Check sheet for the drawn part. Datum: minimum x, y, z corner. Units: mm. A direction names the side the tool comes from. Round coordinates to 2 decimals unless told otherwise and drop trailing zeros. Write each loop counter-clockwise with the first axis right and the second up, starting at its lowest first coordinate (ties: lowest second). Pieces come first, ordered by that corner, then holes. Notation, with made-up numbers: (14, 28.5) -> (37, 28.5) arc R23 ccw to (37, 57.5) -> close; hole circle Ø7 at (-12.75, 62). An arc over 180 degrees is marked (long way). Use CSV: the item, a comma, the result in double quotes.
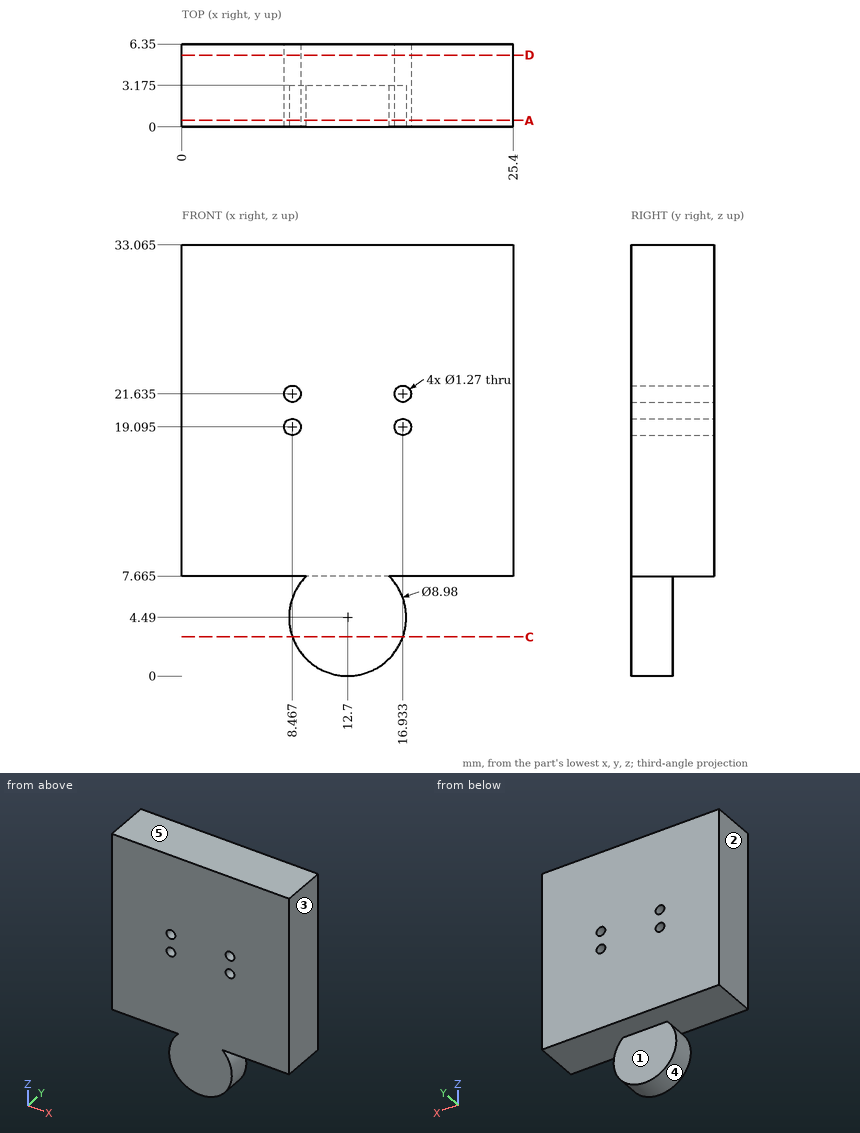
Q1. Mould release check, pull along Z, two halves, no side actions. Record for the marked faces 3, 4 and 5: released by +Z, released by -Z, zero draft, split by the parting line, or undercut.
Filled in:
face 3,"zero draft"
face 4,"undercut"
face 5,"released by +Z"
Q2. Material ranges on L1, parallel to Z at x = 18, y = 3.5 (1 decimal); L2, parallel to Z at x = 10.75, y = 2.25 (1 decimal), recorded low to high.
Filled in:
L1,"7.7 to 33.1"
L2,"0.4 to 33.1"
Q3. Section check A-A (y = 0.5). Record the cut outline in (x, z) (1 decimal), plus the area to 3 significant figures.
Filled in:
outline,"(0, 7.7) -> (9.5, 7.7) arc R4.5 ccw (long way) to (15.9, 7.7) -> (25.4, 7.7) -> (25.4, 33.1) -> (0, 33.1) -> close; hole circle Ø1.3 at (8.5, 19.1); hole circle Ø1.3 at (8.5, 21.6); hole circle Ø1.3 at (16.9, 19.1); hole circle Ø1.3 at (16.9, 21.6)"
area,"698 mm²"
Q4. Section check D-D (y = 5.5). Record the cut outline in (x, z) (1 decimal), plus the area to 3 significant figures.
Filled in:
outline,"(0, 7.7) -> (25.4, 7.7) -> (25.4, 33.1) -> (0, 33.1) -> close; hole circle Ø1.3 at (8.5, 19.1); hole circle Ø1.3 at (8.5, 21.6); hole circle Ø1.3 at (16.9, 19.1); hole circle Ø1.3 at (16.9, 21.6)"
area,"640 mm²"
Q5. Section check C-C (z = 3). Record the cut outline in (x, y) (1 decimal).
Filled in:
outline,"(8.5, 0) -> (16.9, 0) -> (16.9, 3.2) -> (8.5, 3.2) -> close"
Q6. Access from +Z, -Z, +X, -X, +Y, -Y to the whole of each face (thin tool, end or side, straight path). Record for the marked faces 1 and 2.
Filled in:
face 1,"-Z, +X, -X, +Y"
face 2,"+Z, -Z, -X, +Y, -Y"
Q7. Go/stop test with a flat-tipped pin: P1, Ø2.5, axis at x = 12, z = 3, coming from the +Y side (3 decimals). Record where the tip stops, or that it passes through.
Filled in:
P1,"y = 3.175"
